Can you work these out from the model? Positions are in its coordinate system, mm. Coordinates: 2 decimals unless noted, no trailing zeros. Order: outer loops, then holes, each group sorted by start corner. A loop starts at its lowest first (then second) coordinate and runs counter-clockwise, first axis right, second up. Notation, with made-up numbers: (-18, -32.75) -> (18, -32.75) arc R18 cw to (18, -18.75) -> close; hole circle Ø9 at (82.5, -20). An arc over 180 degrees is marked (long way). Answer as a JSON object with one key per item and string values. Group by question number.
(1) For pin 1 (2.5 mm diameter, centred on y = -3, z = -6.5, fed in from +X); pin 2 (3 mm diameter, centred on y = 17, z = -4, fed in from -X); pin 3 (2.5 mm diameter, centred on y = -3, z = -3, fed in from -X), each with a flat end and sliding along its axis, tell me the tip position at first contact or that it passes through.
(2) I want a section at D-D, the plane x = 16.5. List the corners of the cut face in (y, z) for me, plus the area to 3 significant figures.
(3) I need wall thicknesses on line 1 (Y direction, x = 29.5, z = 8.25); line 2 (X direction, y = 6.5, z = 0.25); line 3 (Z direction, x = 58.5, y = 6). Which ranges of each line are inside material? Lowest first, please.
(4) I want a section at A-A, the plane x = 28. List the corners of the cut face in (y, z) for me, plus the area to 3 significant figures.
(5) I want a section at C-C, the plane y = 16. List the corners of the cut face in (x, z) for me.
(6) I want a section at B-B, the plane z = -8. List the corners of the cut face in (x, y) for me, plus the area to 3 significant figures.
from build123d import *

# Parameters (mm, degrees)
EXTRUDE_1_DEPTH = 27
SKETCH_2_W      = 15
SKETCH_2_H      = 8
EXTRUDE_2_DEPTH = 5


with BuildPart() as part:
    # 草图1 → 凸台-拉伸1 (new body)
    with BuildSketch(Plane(origin=(0, 0, 0), x_dir=(1, 0, 0), z_dir=(0, 1, 0))):
        with BuildLine():
            Line((0, 12.15), (55.7, 12.15))
            ThreePointArc((55.7, 12.15), (67.85, 0), (55.7, -12.15))
            Line((55.7, -12.15), (0, -12.15))
            ThreePointArc((0, -12.15), (-12.15, 0), (0, 12.15))
        make_face()
    extrude(amount=EXTRUDE_1_DEPTH)

    # 草图2 → 凸台-拉伸2 (add)
    with BuildSketch(Plane.XZ):
        with Locations((27.85, -4.85)):
            Rectangle(SKETCH_2_W, SKETCH_2_H)
    extrude(amount=EXTRUDE_2_DEPTH)


solid = part.part
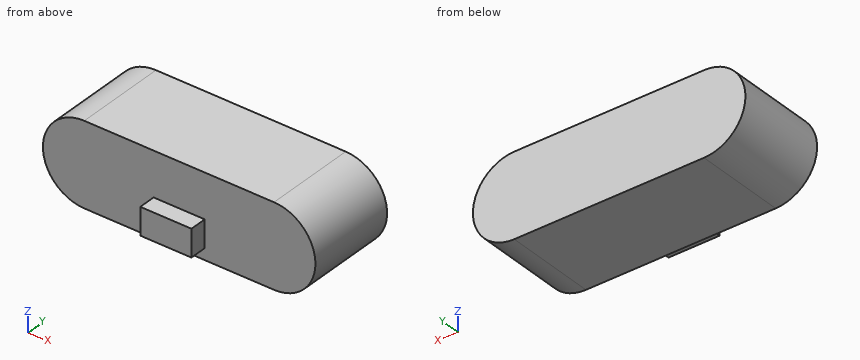
Computed values:
{
 "1": {"pin 1": "stops at x = 35.35", "pin 2": "stops at x = -11.89", "pin 3": "stops at x = 20.35"},
 "2": {"outline": "(0, -12.15) -> (27, -12.15) -> (27, 12.15) -> (0, 12.15) -> close", "area": "656 mm2"},
 "3": {"line 1": "y = 0 to 27", "line 2": "x = -12.15 to 67.85", "line 3": "z = -11.82 to 11.82"},
 "4": {"outline": "(-5, -8.85) -> (0, -8.85) -> (0, -12.15) -> (27, -12.15) -> (27, 12.15) -> (0, 12.15) -> (0, -0.85) -> (-5, -0.85) -> close", "area": "696 mm2"},
 "5": {"outline": "(0, -12.15) -> (55.7, -12.15) arc R12.15 ccw to (55.7, 12.15) -> (0, 12.15) arc R12.15 ccw to start"},
 "6": {"outline": "(-9.14, 0) -> (20.35, 0) -> (20.35, -5) -> (35.35, -5) -> (35.35, 0) -> (64.84, 0) -> (64.84, 27) -> (-9.14, 27) -> close", "area": "2,070 mm2"}
}
